Check sheet for the modelled part. Datum: model origin and axes. Units: mm. Coordinates: 2 decimals unless noted, no trailing zeros. Order: outer loops, then holes, each group sorted by start corner. A loop starts at its lowest first (then second) coordinate and runs counter-clockwise, first axis right, second up.
1. Cross-section at A-A (x = -40). Enter the section's corners in (y, z), then the cut area to 3 significant figures.
2. Thickness scan on line 1 (X direction, y = 0.6, z = -40); line 2 (X direction, y = 1.5, z = -60); line 3 (Z direction, x = -41, y = 0.5). Record the ranges inside material, lowest first.
3. Cross-section at B-B (y = 1.85). Enter the section's corners in (x, z).
4. Gauge pin test, flat ends, axial feed: pin 1 Ø6.5 at (x, z) = (-60, -60) entering from -Y; pin 2 Ø1 at (x, y) = (-52.5, 1.5) entering from +Z. Record the tip position at first contact, or that the pin passes through.
5. Cross-section at C-C (z = -50). Enter the section's corners in (x, y).
6. Cross-section at D-D (x = -55.5). Enter the section's corners in (y, z).
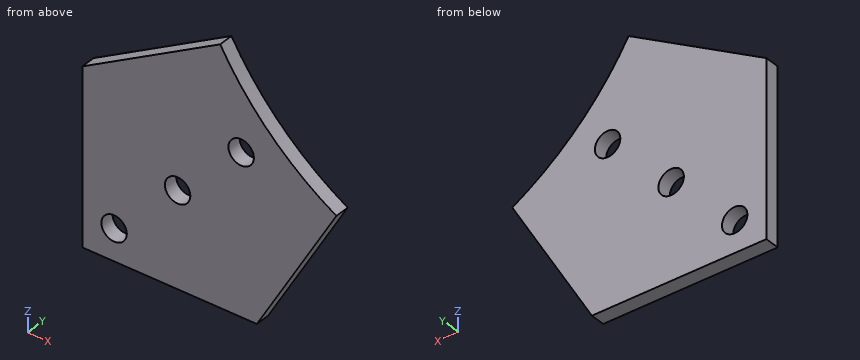
```python
from build123d import *

# Parameters (mm, degrees)
BOSS_EXTRUDE1_DEPTH = 2.3
SKETCH4_R           = 2
SKETCH4_R_2         = 50
CUT_EXTRUDE1_DEPTH  = 92.952650859


with BuildPart() as part:
    # Sketch3 → Boss-Extrude1 (new body)
    with BuildSketch(Plane(origin=(0, 0, 0), x_dir=(1, 0, 0), z_dir=(0, 1, 0))):
        Polygon((-65, 65), (-37.527767497, 65), (-25, 43.301270189), (-43.301270189, 25), (-65, 37.527767497), align=None)
    extrude(amount=BOSS_EXTRUDE1_DEPTH)

    # Sketch4 → Cut-Extrude1 (cut, through all)
    with BuildSketch(Plane(origin=(0, 2.3, 0), x_dir=(1, 0, 0), z_dir=(0, 1, 0))):
        with Locations(Location((-60, 60, 0), (0, 0, 270))):
            Circle(SKETCH4_R)
        with Locations(Location((-50, 50, 0), (0, 0, 270))):
            Circle(SKETCH4_R)
        with Locations(Location((-40, 40, 0), (0, 0, 270))):
            Circle(SKETCH4_R)
        Circle(SKETCH4_R_2)
    extrude(amount=-CUT_EXTRUDE1_DEPTH, mode=Mode.SUBTRACT)


solid = part.part
```
Data:
1. outline: (0, -65) - (2.3, -65) - (2.3, -42) - (0, -42) - close; (0, -38) - (2.3, -38) - (2.3, -30) - (0, -30) - close
1. area: 71.3 mm2
2. line 1: x = -65 to -42, -38 to -30
2. line 2: x = -65 to -62, -58 to -34.64
2. line 3: z = -65 to -41.73, -38.27 to -28.62
3. outline: (-65, -65) - (-37.53, -65) - (-25, -43.3) arc R50 cw to (-43.3, -25) - (-65, -37.53) - close; hole circle Ø4 at (-60, -60); hole circle Ø4 at (-50, -50); hole circle Ø4 at (-40, -40)
4. pin 1: stops at y = 0
4. pin 2: stops at z = -30.02
5. outline: (-65, 0) - (-52, 0) - (-52, 2.3) - (-65, 2.3) - close; (-48, 0) - (-28.87, 0) - (-28.87, 2.3) - (-48, 2.3) - close
6. outline: (0, -65) - (2.3, -65) - (2.3, -32.04) - (0, -32.04) - close
